```python
from build123d import *

# Parameters (mm, degrees)
F0_R     = 2.2225
F0_R_2   = 1.75
F0_W     = 12.7
F0_H     = 7.62
F1_DEPTH = 3.175
F3_DEPTH = 10
F5_DEPTH = 2
F6_R     = 2.54


with BuildPart() as f1:
    # F0 (on Top) → F1 (new body)
    with BuildSketch(Plane.XY):
        with BuildLine():
            Line((40, -25.617377), (40, 25.617377))
            ThreePointArc((40, 25.617377), (0, 47.5), (-40, 25.617377))
            Line((-40, 25.617377), (-40, -25.617377))
            ThreePointArc((-40, -25.617377), (0, -47.5), (40, -25.617377))
        make_face()
        with Locations((-22.225, -37.1475)):
            Circle(F0_R, mode=Mode.SUBTRACT)
        with Locations((-18.75, -17.5)):
            Circle(F0_R_2, mode=Mode.SUBTRACT)
        with Locations((0, -40.31)):
            Rectangle(F0_W, F0_H, mode=Mode.SUBTRACT)
        with Locations((22.225, -37.1475)):
            Circle(F0_R, mode=Mode.SUBTRACT)
        with Locations((18.75, -17.5)):
            Circle(F0_R_2, mode=Mode.SUBTRACT)
        with Locations((-18.75, 17.5)):
            Circle(F0_R_2, mode=Mode.SUBTRACT)
        with Locations((-22.225, 37.1475)):
            Circle(F0_R, mode=Mode.SUBTRACT)
        with Locations((18.75, 17.5)):
            Circle(F0_R_2, mode=Mode.SUBTRACT)
        with Locations((0, 40.31)):
            Rectangle(F0_W, F0_H, mode=Mode.SUBTRACT)
        with Locations((22.225, 37.1475)):
            Circle(F0_R, mode=Mode.SUBTRACT)
    extrude(amount=F1_DEPTH)

    # F2 (on face) → F3 (join)
    with BuildSketch(Plane.XY.offset(3.175)):
        Polygon((-31.5, -24.5), (-31.5, -27), (31.5, -27), (31.5, -24.5), (-29, -24.5), (-29, -5), (-31.5, -5), align=None)
        Polygon((31.5, 24.5), (31.5, 27), (-31.5, 27), (-31.5, 24.5), (-31.5, 5), (-29, 5), (-29, 24.5), align=None)
    extrude(amount=F3_DEPTH)

    # F4 (on face) → F5 (join)
    with BuildSketch(Plane.XY.offset(13.175)):
        Polygon((-31.5, -27), (31.5, -27), (31.5, -19.5), (-24, -19.5), (-24, -5), (-31.5, -5), (-31.5, -19.5), align=None)
        Polygon((-31.5, 14.288086), (-31.5, 5), (-24, 5), (-24, 19.5), (31.5, 19.5), (31.5, 27), (-31.5, 27), (-31.5, 20.743756), (-31.5, 19.5), align=None)
    extrude(amount=-F5_DEPTH)

    # F6
    f6_edges = [f1.edges().sort_by_distance(p)[0] for p in [
        (1.25, -24.5, 11.175),
        (1.25, 24.5, 11.175),
        (-29, -14.75, 11.175),
        (-29, 14.75, 11.175),
    ]]
    fillet(f6_edges, radius=F6_R)


solid = f1.part
```
Read the model definition and answer for the solid it produces. Units are mm, in the model's axes. A direction names the side the tool comes from. Give positions to 0.01 mm unless a question says otherwise; leave off trailing zeros. Write each loop counter-clockwise with the first axis right and the second up, starting at its lowest first coordinate (ties: lowest second). Pieces come first, ordered by that corner, then holes. Notation, with made-up numbers: (18.25, -32) -> (71.25, -32) arc R21 cw to (71.25, -5) -> close; hole circle Ø8 at (20.25, 21). An arc over 180 degrees is marked (long way). Answer in a Markdown table with one row per item.
1) Determine the mould class of faces 1 (the cylindrical face through (20.587, -35.645, 1.565)), 2 (the flat face through (6.35, 40, 2)), 3 (the flat face through (-31.5, 16, 8)), 4 (the flat face through (-7, -21, 13.175)) for opening direction X: released by +X, released by -X, zero draft, split by the parting line, or undercut.
Results list:
| item | result |
|---|---|
| face 1 | undercut |
| face 2 | undercut |
| face 3 | released by -X |
| face 4 | zero draft |
2) Section D-D on y = -7.5 is taken. Give the vertices of the cut face in (x, z) (3 decimals).
Results list:
| item | result |
|---|---|
| outline | (-40, 0) -> (40, 0) -> (40, 3.175) -> (-29, 3.175) -> (-29, 8.635) arc R2.54 cw to (-26.46, 11.175) -> (-24, 11.175) -> (-24, 13.175) -> (-31.5, 13.175) -> (-31.5, 3.175) -> (-40, 3.175) -> close |
3) Straight lines are drawn through the part: line 1 (Y direction, x = 7.5, z = 3.75); line 2 (Y direction, x = -18.75, z = 1.05); line 3 (Y direction, x = -11, z = 12.5). For each, find the intervals that lie inside material, in ascending order. Write a range as [from, to].
Results list:
| item | result |
|---|---|
| line 1 | [-27, -24.5], [24.5, 27] |
| line 2 | [-43.64, -19.25], [-15.75, 15.75], [19.25, 43.64] |
| line 3 | [-27, -19.5], [19.5, 27] |
4) Section A-A on y = -17.5 is taken. Give the vertices of the cut face in (x, z) (3 decimals), plus the area to 3 significant figures.
Results list:
| item | result |
|---|---|
| outline | (-40, 0) -> (-20.5, 0) -> (-20.5, 3.175) -> (-29, 3.175) -> (-29, 8.635) arc R2.54 cw to (-26.46, 11.175) -> (-24, 11.175) -> (-24, 13.175) -> (-31.5, 13.175) -> (-31.5, 3.175) -> (-40, 3.175) -> close; (-17, 0) -> (17, 0) -> (17, 3.175) -> (-17, 3.175) -> close; (20.5, 0) -> (40, 0) -> (40, 3.175) -> (20.5, 3.175) -> close |
| area | 268 mm^2 |
5) Each of these flat-tipped pins is pushed along its axis until it touches: pin 1 Ø3 at (y, z) = (-8.5, 9) entering from +X; pin 2 Ø4 at (x, z) = (-24.5, 8.5) entering from -Y; pin 3 Ø2.5 at (x, z) = (-2.5, 2) entering from +Y. Where does it stop, or does it pass through?
Results list:
| item | result |
|---|---|
| pin 1 | x = -28.18 |
| pin 2 | y = -27 |
| pin 3 | y = 47.48 |
6) Section B-B on x = 0 is taken. Give the vertices of the cut face in (y, z) (3 decimals), plus the area to 3 significant figures.
Results list:
| item | result |
|---|---|
| outline | (-47.5, 0) -> (-44.12, 0) -> (-44.12, 3.175) -> (-47.5, 3.175) -> close; (-36.5, 0) -> (36.5, 0) -> (36.5, 3.175) -> (27, 3.175) -> (27, 13.175) -> (19.5, 13.175) -> (19.5, 11.175) -> (21.96, 11.175) arc R2.54 cw to (24.5, 8.635) -> (24.5, 3.175) -> (-24.5, 3.175) -> (-24.5, 8.635) arc R2.54 cw to (-21.96, 11.175) -> (-19.5, 11.175) -> (-19.5, 13.175) -> (-27, 13.175) -> (-27, 3.175) -> (-36.5, 3.175) -> close; (44.12, 0) -> (47.5, 0) -> (47.5, 3.175) -> (44.12, 3.175) -> close |
| area | 326 mm^2 |
7) A tool of negligible diameter and unlimited length cuts with its end or side. For faces 5 (the flat face through (-6.35, -40, 2)), 6 (the flat face through (-2, -20, 11.175)), 7 (the flat face through (31.5, 25, 9)), from which of +Z, -Z, +X, -X, +Y, -Y can it reach the whole face along a straight path? Write none if from no direction.
Results list:
| item | result |
|---|---|
| face 5 | +Z, -Z |
| face 6 | +X |
| face 7 | +Z, +X, +Y, -Y |
8) Section C-C on z = 4.75 is taken. Give the vertices of the cut face in (x, y).
Results list:
| item | result |
|---|---|
| outline | (-31.5, -27) -> (31.5, -27) -> (31.5, -24.5) -> (-29, -24.5) -> (-29, -5) -> (-31.5, -5) -> close; (-31.5, 5) -> (-29, 5) -> (-29, 24.5) -> (31.5, 24.5) -> (31.5, 27) -> (-31.5, 27) -> close |
